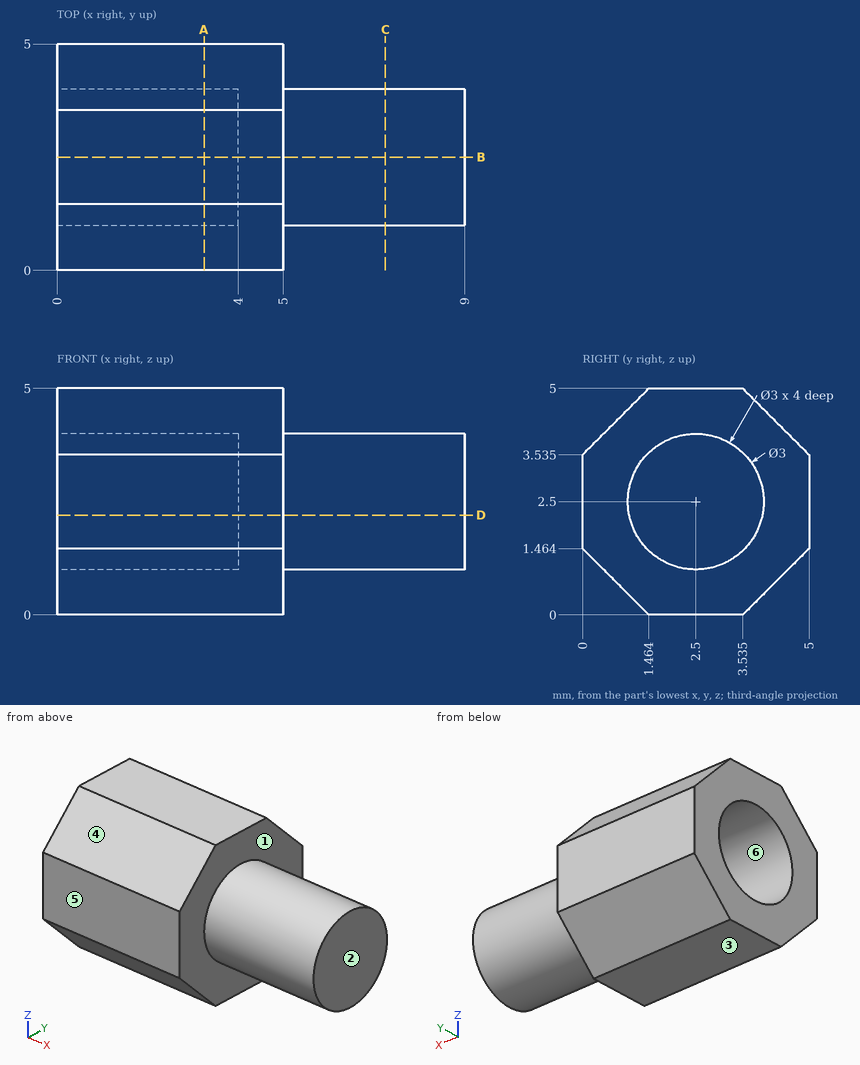
Geometry check sheet. Reference: drawing and pictorial views, mm from the part's lowest x, y, z. A direction names the side the tool comes from. Give positions to 0.01 mm unless a question says otherwise; leave off trailing zeros. Order: outer loops, then holes, each group sorted by start corner. A loop starts at its lowest first (then second) coordinate and runs counter-clockwise, first axis right, second up. Notation, with made-up numbers: M 52.25,-34.5 L 77.25,-34.5 A10 cw 77.25,-15.5 Z; hole C -22,-29 d2. An arc over 180 degrees is marked long. Return JSON: item names as keys, results as strings. Group by question number.
1) Scan lines: line 1 (Z direction, x = 2.65, y = 2.5); line 2 (X direction, y = 2.4, z = 0.6); line 3 (Y direction, x = 3.5, z = 1.5). Record each from-to range of solid material in increasing order.
2) Section check D-D on z = 2.2. Record the cut outline in (x, y).
3) Mould release check, pull along Z, two halves, no side actions. Record for the marked faces 3, 4, 5 and 6: pulls with the +Z half, pulls with the -Z half, needs draft (parallel to the pull), parting line crosses it, or undercut.
4) Section check A-A on x = 3.25. Record the cut outline in (y, z) (1 decimal).
5) Access from +Z, -Z, +X, -X, +Y, -Y to the whole of each face (thin tool, end or side, straight path). Record for the marked faces 1 and 2.
6) Section check C-C on x = 7.25. Record the cut outline in (y, z).
7) Section check B-B on y = 2.5. Record the cut outline in (x, z), and give its area (3 significant figures).
8) Go/stop test with a flat-tipped pin: pin 1 Ø2 at (x, y) = (6.5, 3.5) entering from +Z. Record where the tip stops, or that it passes through.
Answer block:
{
 "1": {"line 1": "z = 0 to 1, 4 to 5", "line 2": "x = 0 to 5", "line 3": "y = 0 to 1.38, 3.62 to 5"},
 "2": {"outline": "M 0,0 L 5,0 L 5,1.03 L 9,1.03 L 9,3.97 L 5,3.97 L 5,5 L 0,5 L 0,3.97 L 4,3.97 L 4,1.03 L 0,1.03 Z"},
 "3": {"face 3": "pulls with the -Z half", "face 4": "pulls with the +Z half", "face 5": "needs draft", "face 6": "undercut"},
 "4": {"outline": "M 0,1.5 L 1.5,0 L 3.5,0 L 5,1.5 L 5,3.5 L 3.5,5 L 1.5,5 L 0,3.5 Z; hole C 2.5,2.5 d3"},
 "5": {"face 1": "+X", "face 2": "+Z, -Z, +X, +Y, -Y"},
 "6": {"outline": "C 2.5,2.5 d3"},
 "7": {"outline": "M 0,0 L 5,0 L 5,1 L 9,1 L 9,4 L 5,4 L 5,5 L 0,5 L 0,4 L 4,4 L 4,1 L 0,1 Z", "area": "25.0 mm^2"},
 "8": {"pin 1": "stops at z = 4"}
}
